Work out the finished part from the listing and answer in its coordinate system (mm). A direction names the side the tool comes from. Round coordinates to 2 decimals unless told otherwise and drop trailing zeros. Order: outer loops, then holes, each group sorted by start corner. A loop starts at its lowest first (then second) coordinate and runs counter-clockwise, first axis right, second up. Notation, with made-up numbers: (-11.5, 45.25) - (31.5, 45.25) arc R20 ccw to (31.5, 50.25) - close; hole circle Ø7 at (70, 56). An arc over 180 degrees is marked (long way). Use CSV: the item, a comma, the result in double quotes.
Autodesk Inventor part; units mm, degrees
ref_plane "YZ Plane" through (0, 0, 0) normal (1, 0, 0) x (0, 1, 0)
ref_plane "XZ Plane" through (0, 0, 0) normal (0, 1, 0) x (-1, 0, 0)
ref_plane "XY Plane" through (0, 0, 0) normal (0, 0, 1) x (1, 0, 0)
sketch "Sketch1" plane through (0, 0, 0) normal (0, 1, 0) x (-1, 0, 0)
  circle A0 centre (0, 0) radius 17.325
  circle A1 centre (0, 0) radius 3
  dimension "d0" = 34.65
  dimension "d1" = 6
extrude "Extrusion1" add sketch "Sketch1" along normal blind 4.1
sketch "Sketch2" plane through (0, 4.1, 0) normal (0, 1, 0) x (1, 0, 0)
  circle A0 centre (0, 0) radius 3
  circle A1 centre (0, 0) radius 17.325
  circle A2 centre (0, 0) radius 14.5
  dimension "d4" = 29
extrude "Extrusion2" add sketch "Sketch2" along normal blind 1 contours A2
sketch "Sketch3" plane through (0, 5.1, 0) normal (0, 1, 0) x (1, 0, 0)
  circle A0 centre (0, 0) radius 3
extrude "Extrusion3" add sketch "Sketch3" against normal blind 1
sketch "Sketch4" plane through (0, 5.1, 0) normal (0, 1, 0) x (1, 0, 0)
  circle A0 centre (0, 0) radius 14.5
  circle A1 centre (0, 0) radius 5
  dimension "d9" = 10
extrude "Extrusion4" add sketch "Sketch4" along normal blind 3.8 contours A1
sketch "Sketch5" plane through (0, 8.9, 0) normal (0, 1, 0) x (1, 0, 0)
  circle A0 centre (0, 0) radius 5
  circle A1 centre (0, 0) radius 3
  dimension "d12" = 6
extrude "Extrusion5" cut sketch "Sketch5" against normal blind 3.8 contours A1
properties part number "kolecko_servo(2)"
(1) Find section B-B (x = 0). Determine the outline of the cut face in (y, z) (3 decimals).
Findings below:
outline,"(0, -17.325) - (4.1, -17.325) - (4.1, -14.5) - (5.1, -14.5) - (5.1, -5) - (8.9, -5) - (8.9, -3) - (5.1, -3) - (5.1, 3) - (8.9, 3) - (8.9, 5) - (5.1, 5) - (5.1, 14.5) - (4.1, 14.5) - (4.1, 17.325) - (0, 17.325) - (0, 3) - (4.1, 3) - (4.1, -3) - (0, -3) - close"
(2) Find the intervals of material crossed by L1, parallel to X at y = 7.65, z = 0; L2, parallel to Z at x = 0, y = 3.05 (3 decimals), in increasing order. Write a range as from..to.
Findings below:
L1,"x = -5..-3, 3..5"
L2,"z = -17.325..-3, 3..17.325"
(3) Find section C-C (z = 0). Determine the outline of the cut face in (x, y) (3 decimals), and give its area (3 significant figures).
Findings below:
outline,"(-17.325, 0) - (-3, 0) - (-3, 4.1) - (3, 4.1) - (3, 0) - (17.325, 0) - (17.325, 4.1) - (14.5, 4.1) - (14.5, 5.1) - (5, 5.1) - (5, 8.9) - (3, 8.9) - (3, 5.1) - (-3, 5.1) - (-3, 8.9) - (-5, 8.9) - (-5, 5.1) - (-14.5, 5.1) - (-14.5, 4.1) - (-17.325, 4.1) - close"
area,"162 mm²"
(4) Find section A-A (y = 1.75). Determine the outline of the cut face in (x, z) (3 decimals).
Findings below:
outline,"circle Ø34.65 at (0, 0); hole circle Ø6 at (0, 0)"
(5) Find section D-D (x = -14). Determine the outline of the cut face in (y, z), and give its area (3 significant figures).
Findings below:
outline,"(0, -10.21) - (4.1, -10.21) - (4.1, -3.77) - (5.1, -3.77) - (5.1, 3.77) - (4.1, 3.77) - (4.1, 10.21) - (0, 10.21) - close"
area,"91.2 mm²"
(6) Each of these flat-tipped pins is pushed along its axis until it touches: pin 1 (3.5 mm diameter, centred on x = 0, z = 0, fed in from +Y); pin 2 (5.5 mm diameter, centred on x = 0, z = 0, fed in from -Y); pin 3 (1.5 mm diameter, centred on y = 3.5, z = -10, fed in from +X). Where does it stop, or does it pass through?
Findings below:
pin 1,"stops at y = 5.1"
pin 2,"stops at y = 4.1"
pin 3,"stops at x = 14.65"
(7) The mould has two halves that part along Z. Classify faces 1 (the cylindrical face through (-1.08, 6.97, -4.88)), 2 (the cylindrical face through (3, 2, 0)), 3 (the flat face through (9.1, 4.1, -11.5)): released by +Z, released by -Z, zero draft, split by the parting line, or undercut.
Findings below:
face 1,"split by the parting line"
face 2,"undercut"
face 3,"zero draft"
(8) For faces 4 (the flat face through (-4, 0, 0)), 5 (the cylindrical face through (-3, 7, 0)), 6 (the flat face through (0, 4.1, 0)), determine the directions among +Z, -Z, +X, -X, +Y, -Y from which every point of the face is accessible in a straight line to the end or side of a thin tool.
Findings below:
face 4,"+Z, -Z, +X, -X, -Y"
face 5,"+Y"
face 6,"-Y"
